```python
from build123d import *

# Parameters (mm, degrees)
SKETCH_1_W          = 4
SKETCH_1_H          = 6
SKETCH_1_R          = 1
EXTRUDE_1_DEPTH     = 6
SKETCH_2_W          = 2
SKETCH_2_H          = 1
CUT_EXTRUDE_1_DEPTH = 8.810249676


with BuildPart() as part:
    # 草图1 → 凸台-拉伸1 (new body)
    with BuildSketch(Plane.XY):
        Rectangle(SKETCH_1_W, SKETCH_1_H)
        Circle(SKETCH_1_R, mode=Mode.SUBTRACT)
    extrude(amount=EXTRUDE_1_DEPTH)

    # 草图2 → 切除-拉伸1 (cut, through all)
    with BuildSketch(Plane(origin=(2, 0, 0), x_dir=(0, 0, -1), z_dir=(1, 0, 0))):
        with Locations((-3, 2.5)):
            Rectangle(SKETCH_2_W, SKETCH_2_H)
        with Locations((-3, -2.5)):
            Rectangle(SKETCH_2_W, SKETCH_2_H)
    extrude(amount=-CUT_EXTRUDE_1_DEPTH, mode=Mode.SUBTRACT)


solid = part.part
```
Source: CAD feature listing. Evaluate the final solid. Frame: model axes, mm. A direction names the side the tool comes from. Coordinates: 2 decimals unless noted, no trailing zeros. Loops run counter-clockwise (first coordinate to the right, second up) from the corner with the lowest first, then second, coordinate; pieces in that order, holes last. Notation, with made-up numbers: M -3.75,16.5 L 0.25,16.5 A20 cw 0.25,53.5 Z; hole C 80.25,-3.5 d2. An arc over 180 degrees is marked long. Put each result on its own line as item: value. Start each with the question number.
1) Cut plane C-C on z = 3. Return the cut outline in (x, y), then the cut area to 3 significant figures.
2) Contact query for flat-ended pins moving along their axis: pin 1 Ø1 at (x, z) = (-0.5, 3) entering from +Y; pin 2 Ø0.6 at (x, z) = (0.5, 3.5) entering from -Y. Output: stop coordinate, or through.
3) Cut plane D-D on x = -1.7. Return the cut outline in (y, z), then the cut area to 3 significant figures.
4) Reachability of faces 1 (the face through (0, 2, 3)), 2 (the face through (0, -2.5, 2)), 3 (the face through (0, 3, 1)) from +Z, -Z, +X, -X, +Y, -Y: full face, straight path, thin tool, end or side. Return the list, or none.
5) Ray query, L1, parallel to Z at x = -1.4, y = -2.1; L2, parallel to Y at x = 0, z = 1.5; L3, parallel to Y at x = 0, z = 2.3. Return the intervals inside material, ascending. Write a range as from..to.
6) Cut plane B-B on y = 2.3. Return the cut outline in (x, z), then the cut area to 3 significant figures.
7) Pull-direction query (Z, two-part tool) for faces 4 (the face through (2, 0, 3)), 5 (the face through (0, 2.5, 4)), 6 (the face through (-1, 1, 6)); classes: pulls with the +Z half, pulls with the -Z half, needs draft (parallel to the pull), parting line crosses it, or undercut.
8) Cut plane A-A on x = 0. Return the cut outline in (y, z), then the cut area to 3 significant figures.
The answers:
1. outline: M -2,-2 L 2,-2 L 2,2 L -2,2 Z; hole C 0,0 d2
1. area: 12.9 mm²
2. pin 1: stops at y = 2
2. pin 2: stops at y = -2
3. outline: M -3,0 L 3,0 L 3,2 L 2,2 L 2,4 L 3,4 L 3,6 L -3,6 L -3,4 L -2,4 L -2,2 L -3,2 Z
3. area: 32.0 mm²
4. face 1: +X, -X, +Y
4. face 2: +X, -X, -Y
4. face 3: +Z, -Z, +X, -X, +Y
5. L1: z = 0..2, 4..6
5. L2: y = -3..-1, 1..3
5. L3: y = -2..-1, 1..2
6. outline: M -2,0 L 2,0 L 2,2 L -2,2 Z; M -2,4 L 2,4 L 2,6 L -2,6 Z
6. area: 16.0 mm²
7. face 4: needs draft
7. face 5: undercut
7. face 6: pulls with the +Z half
8. outline: M -3,0 L -1,0 L -1,6 L -3,6 L -3,4 L -2,4 L -2,2 L -3,2 Z; M 1,0 L 3,0 L 3,2 L 2,2 L 2,4 L 3,4 L 3,6 L 1,6 Z
8. area: 20.0 mm²
